Answer from the drawing. Dimensions are ordinates in mm from the lowest x, y and z of the part. Give positions to 0.01 mm unless a question says otherwise; leave off trailing zeros. Write each loop counter-clockwise with the first axis right and the second up, starting at its lowest first coordinate (ties: lowest second). Pieces come first, ordered by that corner, then holes. Notation, with made-up numbers: (85.5, 28.25) -> (95.5, 28.25) arc R16 ccw to (95.5, 59.25) -> close; hole circle Ø1 at (56.25, 65). An arc over 180 degrees is marked (long way). Use a Markdown table: item, result. Add a question column.
Q1. Section B-B, the plane y = 11.43 is taken. Give the vertices of the cut face in (x, z) (3 decimals), plus the area to 3 significant figures.
Q2. Section C-C, the plane z = 0.9 is taken. Give the vertices of the cut face in (x, y) (3 decimals).
Q3. For a pull along X with two mould halves and no side action, classify the marked faces 1, 2 and 3 as pulls with the +X half, pulls with the -X half, needs draft (parallel to the pull), parting line crosses it, or undercut.
Q4. Consider line 1 (Y direction, x = 11.43, z = 2); line 2 (X direction, y = 10, z = 1.7); line 3 (X direction, y = 8, z = 1.5). Determine where each line is inside the solid, lowest interval first.
Q5. Each of these flat-tipped pins is pushed along its axis until it touches: pin 1 Ø1 at (x, z) = (7, 0.5) entering from +Y; pin 2 Ø5 at (x, y) = (13.5, 19) entering from -Z; pin 3 Ø1.5 at (x, z) = (3.5, 2) entering from -Y. Where does it stop, or does it pass through?
Q6. Section A-A, the plane x = 11.43 is taken. Give the vertices of the cut face in (y, z) (3 decimals), plus the area to 3 significant figures.
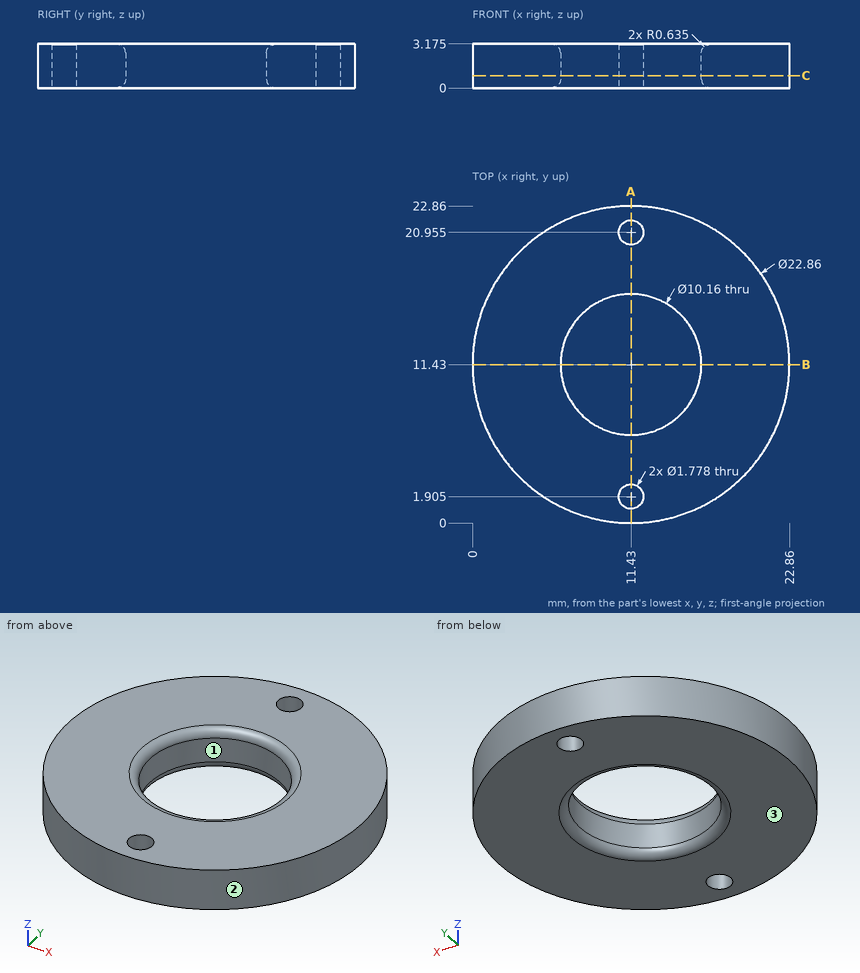
Result set:
| question | item | result |
|---|---|---|
| 1 | outline | (0, 0) -> (5.715, 0) arc R0.635 ccw to (6.35, 0.635) -> (6.35, 2.54) arc R0.635 ccw to (5.715, 3.175) -> (0, 3.175) -> close; (16.51, 0.635) arc R0.635 ccw to (17.145, 0) -> (22.86, 0) -> (22.86, 3.175) -> (17.145, 3.175) arc R0.635 ccw to (16.51, 2.54) -> close |
| 1 | area | 40.0 mm2 |
| 2 | outline | circle Ø22.86 at (11.43, 11.43); hole circle Ø10.16 at (11.43, 11.43); hole circle Ø1.778 at (11.43, 1.905); hole circle Ø1.778 at (11.43, 20.955) |
| 3 | face 1 | undercut |
| 3 | face 2 | parting line crosses it |
| 3 | face 3 | needs draft |
| 4 | line 1 | y = 0 to 1.02, 2.79 to 6.35, 16.51 to 20.07, 21.84 to 22.86 |
| 4 | line 2 | x = 0.09 to 6.56, 16.3 to 22.77 |
| 4 | line 3 | x = 0.53 to 7.68, 15.18 to 22.33 |
| 5 | pin 1 | stops at y = 22.16 |
| 5 | pin 2 | stops at z = 0 |
| 5 | pin 3 | stops at y = 2.54 |
| 6 | outline | (0, 0) -> (1.016, 0) -> (1.016, 3.175) -> (0, 3.175) -> close; (2.794, 0) -> (5.715, 0) arc R0.635 ccw to (6.35, 0.635) -> (6.35, 2.54) arc R0.635 ccw to (5.715, 3.175) -> (2.794, 3.175) -> close; (16.51, 0.635) arc R0.635 ccw to (17.145, 0) -> (20.066, 0) -> (20.066, 3.175) -> (17.145, 3.175) arc R0.635 ccw to (16.51, 2.54) -> close; (21.844, 0) -> (22.86, 0) -> (22.86, 3.175) -> (21.844, 3.175) -> close |
| 6 | area | 28.7 mm2 |
